Work out the finished part from the listing and answer in its coordinate system (mm). Face numbers are marked on the shaded views. Round coordinates to 2 decimals unless told otherwise and drop trailing zeros. Write each loop counter-clockwise with the first axis right and the second up, starting at its lowest first coordinate (ties: lowest second). Pieces come first, ordered by that corner, then holes. Notation, with made-up numbers: M 77.25,-37 L 128.25,-37 A10 ccw 128.25,-26 Z; hole C 23.25,50 d1. An arc over 180 degrees is marked long. Answer in a Markdown table with one row per item.
```python
from build123d import *

# Parameters (mm, degrees)
SKETCH1_R           = 33.75
BOSS_EXTRUDE1_DEPTH = 7.5
SKETCH2_R           = 2.6
CUT_EXTRUDE1_DEPTH  = 2.5
SKETCH3_R           = 23
CUT_EXTRUDE2_DEPTH  = 49.315370225
SKETCH4_R           = 25
CUT_EXTRUDE3_DEPTH  = 5


with BuildPart() as part:
    # Sketch1 → Boss-Extrude1 (new body)
    with BuildSketch(Plane(origin=(0, 0, 0), x_dir=(1, 0, 0), z_dir=(0, 1, 0))):
        with Locations(Location((0, 0, 0), (0, 0, 270))):
            Circle(SKETCH1_R)
    extrude(amount=BOSS_EXTRUDE1_DEPTH)

    # Sketch2 → Cut-Extrude1 (cut)
    with BuildSketch(Plane.XZ):
        with Locations(Location((-30, 0, 0), (0, 0, 270))):
            Circle(SKETCH2_R)
        with Locations(Location((30, 0, 0), (0, 0, 90))):
            Circle(SKETCH2_R)
        with Locations(Location((0, -30, 0), (0, 0, 90))):
            Circle(SKETCH2_R)
        with Locations(Location((0, 30, 0), (0, 0, 270))):
            Circle(SKETCH2_R)
    extrude(amount=-CUT_EXTRUDE1_DEPTH, mode=Mode.SUBTRACT)

    # Sketch3 → Cut-Extrude2 (cut, through all)
    with BuildSketch(Plane(origin=(0, 7.5, 0), x_dir=(1, 0, 0), z_dir=(0, 1, 0))):
        with Locations(Location((0, 0, 0), (0, 0, 270))):
            Circle(SKETCH3_R)
    extrude(amount=-CUT_EXTRUDE2_DEPTH, mode=Mode.SUBTRACT)

    # Sketch4 → Cut-Extrude3 (cut)
    with BuildSketch(Plane(origin=(0, 7.5, 0), x_dir=(1, 0, 0), z_dir=(0, 1, 0))):
        with Locations(Location((0, 0, 0), (0, 0, 270))):
            Circle(SKETCH4_R)
    extrude(amount=-CUT_EXTRUDE3_DEPTH, mode=Mode.SUBTRACT)


solid = part.part
```
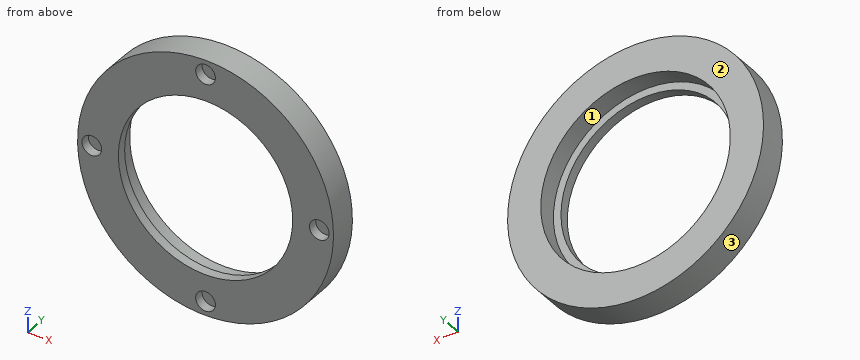
1. Given pin 1 (1.5 mm diameter, centred on x = -16, y = 5.5, fed in from -Z); pin 2 (8 mm diameter, centred on x = -16, z = 8.5, fed in from +Y); pin 3 (1.5 mm diameter, centred on y = 5, z = 2.5, fed in from +X); pin 4 (3 mm diameter, centred on x = -22.5, y = 4, fed in from -Z), each flat-ended and moving along its own axis, determine where each tip first touches the part or whether it passes through.
Calculated:
| item | result |
|---|---|
| pin 1 | stops at z = -30.11 |
| pin 2 | passes through |
| pin 3 | stops at x = 33.7 |
| pin 4 | stops at z = -26.42 |
2. The part is cut by section D-D (x = 30). Determine the outline of the cut face in (y, z).
Calculated:
| item | result |
|---|---|
| outline | M 0,-15.46 L 7.5,-15.46 L 7.5,15.46 L 0,15.46 L 0,2.6 L 2.5,2.6 L 2.5,-2.6 L 0,-2.6 Z |
3. The part is cut by section A-A (x = 0). Determine the outline of the cut face in (y, z).
Calculated:
| item | result |
|---|---|
| outline | M 0,-33.75 L 7.5,-33.75 L 7.5,-25 L 2.5,-25 L 2.5,-23 L 0,-23 L 0,-27.4 L 2.5,-27.4 L 2.5,-32.6 L 0,-32.6 Z; M 0,23 L 2.5,23 L 2.5,25 L 7.5,25 L 7.5,33.75 L 0,33.75 L 0,32.6 L 2.5,32.6 L 2.5,27.4 L 0,27.4 Z |
4. The part is cut by section B-B (z = -13). Determine the outline of the cut face in (x, y).
Calculated:
| item | result |
|---|---|
| outline | M -31.15,0 L -18.97,0 L -18.97,2.5 L -21.35,2.5 L -21.35,7.5 L -31.15,7.5 Z; M 18.97,0 L 31.15,0 L 31.15,7.5 L 21.35,7.5 L 21.35,2.5 L 18.97,2.5 Z |
5. Consider line 1 along X through (y, z) = (2, 0); line 2 along Z through (x, y) = (1, 2.25); line 3 along Z through (x, y) = (30, 0.8). Determine where each line is inside the solid, lowest interval first. Write a range as from..to.
Calculated:
| item | result |
|---|---|
| line 1 | x = -33.75..-32.6, -27.4..-23, 23..27.4, 32.6..33.75 |
| line 2 | z = -33.74..-32.4, -27.6..-22.98, 22.98..27.6, 32.4..33.74 |
| line 3 | z = -15.46..-2.6, 2.6..15.46 |
6. Determine the mould class of the marked faces 1, 2 and 3 for opening direction Z: released by +Z, released by -Z, zero draft, split by the parting line, or undercut.
Calculated:
| item | result |
|---|---|
| face 1 | undercut |
| face 2 | zero draft |
| face 3 | split by the parting line |
7. The part is cut by section C-C (y = 4.25). Determine the outline of the cut face in (x, z), plus the area to 3 significant figures.
Calculated:
| item | result |
|---|---|
| outline | C 0,0 d67.5; hole C 0,0 d50 |
| area | 1,610 mm² |
